Could you check a few things on this model? Use its own coordinates, in mm. A direction names the side the tool comes from. Round coordinates to 2 decimals unless told otherwise and drop trailing zeros. Write each loop counter-clockwise with the first axis right and the second up, starting at its lowest first coordinate (ties: lowest second). Pieces come first, ordered by that corner, then holes. Notation, with made-up numbers: (74, 86) - (96, 86) arc R34 ccw to (96, 117) - close; hole circle Ø6 at (28, 82). An arc over 180 degrees is marked (long way). Put each result on its own line as item: value.
Autodesk Inventor part; units mm, degrees
ref_plane "YZ Plane" through (0, 0, 0) normal (1, 0, 0) x (0, 1, 0)
ref_plane "XZ Plane" through (0, 0, 0) normal (0, 1, 0) x (-1, 0, 0)
ref_plane "XY Plane" through (0, 0, 0) normal (0, 0, 1) x (1, 0, 0)
sketch "スケッチ1" plane through (0, 0, 0) normal (0, 0, 1) x (1, 0, 0)
  circle A0 centre (0, 0) radius 46
  line L0 (0, 54.251) -> (0, -59.4354)
  line L1 (-57.6108, 0) -> (60.5194, 0)
  circle A1 centre (0, 0) radius 48.5
  line L2 (0, 0) -> (-23.2819, 56.2075)
  line L3 (-23.2819, 56.2075) -> (0, 0)
  line L4 (0, 0) -> (23.2706, 56.1801)
  point P0 (-17.6034, 42.4985)
  point P1 (17.6034, 42.4985)
  point P2 (-42.4985, -17.6034)
  point P3 (-42.4985, 17.6034)
  point P4 (17.6034, -42.4985)
  point P5 (-17.6034, -42.4985)
  point P6 (42.4985, 17.6034)
  point P7 (42.4985, -17.6034)
  dimension "d0" = 92
  dimension "d1" = 97
  dimension "d2" = 45
  dimension "d3" = 22.5
  dimension "d6" = 360
extrude "押し出し1" add sketch "スケッチ1" along normal blind 24
sketch "スケッチ2" plane through (0, 0, 24) normal (0, 0, 1) x (1, 0, 0)
  line L0 (0, 68.9903) -> (0, -65.3185)
  circle A0 centre (0, 0) radius 46
  line L1 (0, 0) -> (-21.3879, 51.6351)
  line L2 (-21.3879, 51.6351) -> (0, 0)
  line L3 (0, 0) -> (19.8653, 47.959)
  point P0 (-17.6034, 42.4985)
  point P1 (17.6034, 42.4985)
  point P2 (-42.4985, -17.6034)
  point P3 (-42.4985, 17.6034)
  point P4 (17.6034, -42.4985)
  point P5 (-17.6034, -42.4985)
  point P6 (42.4985, 17.6034)
  point P7 (42.4985, -17.6034)
  dimension "d10" = 92
  dimension "d11" = 45
  dimension "d12" = 22.5
  dimension "d15" = 360
hole "穴1" at (-17.6034, 42.4985, 24) at (17.6034, 42.4985, 24) at (-42.4985, -17.6034, 24) at (-42.4985, 17.6034, 24) at (17.6034, -42.4985, 24) at (-17.6034, -42.4985, 24) at (42.4985, 17.6034, 24) at (42.4985, -17.6034, 24) direction (0, 0, -1) diameter 2.459 end through all
sketch "スケッチ3" plane through (0, 0, 24) normal (0, 0, 1) x (1, 0, 0)
  circle A0 centre (0, 0) radius 30
  dimension "d24" = 60
extrude "押し出し2" add sketch "スケッチ3" along normal blind 1
sketch "スケッチ4" plane through (0, 0, 25) normal (0, 0, 1) x (1, 0, 0)
  circle A0 centre (0, 0) radius 25
  dimension "d27" = 50
extrude "押し出し3" add sketch "スケッチ4" along normal blind 3.8
sketch "スケッチ5" plane through (0, 0, 28.8) normal (0, 0, 1) x (1, 0, 0)
  circle A0 centre (0, 0) radius 17
  dimension "d30" = 34
extrude "押し出し4" add sketch "スケッチ5" along normal blind 0.7
sketch "スケッチ6" plane through (0, 0, 29.5) normal (0, 0, 1) x (1, 0, 0)
  line L0 (0, 40.5289) -> (0, -45.0936)
  line L1 (-34.581, 0) -> (35.411, 0)
  point P0 (0, 0)
properties part number "GIM8108-8"
(1) I'm going to push flat-ended pins straight in: pin 1 (12 mm diameter, centred on x = 22.5, z = 20.5, fed in from -Y); pin 2 (1 mm diameter, centred on y = -22, z = 16.5, fed in from -X); pin 3 (8 mm diameter, centred on x = 11.5, y = 21.5, fed in from +Z). Where does each tip first touch, or does it pass through?
Values found:
pin 1: stops at y = -45.61
pin 2: stops at x = -43.47
pin 3: stops at z = 28.8
(2) Imagine slicing it at D-D, the plane y = -22. List the corners of the cut face in (x, z) for me.
Values found:
outline: (-43.22, 0) - (43.22, 0) - (43.22, 24) - (20.4, 24) - (20.4, 25) - (11.87, 25) - (11.87, 28.8) - (-11.87, 28.8) - (-11.87, 25) - (-20.4, 25) - (-20.4, 24) - (-43.22, 24) - close
(3) Imagine slicing it at A-A, the plane x = 0. List the corners of the cut face in (y, z) for me.
Values found:
outline: (-48.5, 0) - (48.5, 0) - (48.5, 24) - (30, 24) - (30, 25) - (25, 25) - (25, 28.8) - (17, 28.8) - (17, 29.5) - (-17, 29.5) - (-17, 28.8) - (-25, 28.8) - (-25, 25) - (-30, 25) - (-30, 24) - (-48.5, 24) - close
(4) Imagine slicing it at B-B, the plane z = 15.5. Give the number of separate pieces and of enclosed holes in the cut face, then the cut area to 3 significant figures.
Values found:
separate pieces: 1
enclosed holes: 8
area: 7,350 mm^2
(5) If we mould it in two halves opening along Y, with no side actions, what happens to faces 1 (the face through (43.25, -16.63, 11.83)), 2 (the face through (22.38, 43.028, 11.832)), 3 (the face through (-1, 1, 0))? For each: pulls with the +Y half, pulls with the -Y half, needs draft (parallel to the pull), parting line crosses it, or undercut.
Values found:
face 1: undercut
face 2: parting line crosses it
face 3: needs draft
(6) Please list where these lines run through material, in increasing order: probe 1 along X at (y, z) = (42, 6.5); probe 2 along X at (y, z) = (42.5, 6.25); probe 3 along Y at (x, z) = (43, 12.25). Write a range as from..to.
Values found:
probe 1: x = -24.25..-18.73, -16.48..16.48, 18.73..24.25
probe 2: x = -23.37..-18.83, -16.37..16.37, 18.83..23.37
probe 3: y = -22.43..-18.73, -16.48..16.48, 18.73..22.43
(7) For faces 4 (the face through (-41.75, -16.63, 11.83)), 5 (the face through (-7, 25, 25)), which set-ups out of +Z, -Z, +X, -X, +Y, -Y let a thin tool reach every point of the face, with its end or its side?
Values found:
face 4: +Z, -Z
face 5: +Z
